Input: dimensioned drawing with shaded views. Units: mm. Origin: part minimum x, y, z. A direction names the side the tool comes from. Coordinates: 2 decimals unless noted, no trailing zeros. Order: outer loops, then holes, each group sorted by start corner. A loop starts at its lowest first (then second) coordinate and runs counter-clockwise, first axis right, second up. Notation, with made-up numbers: (57.5, 5) -> (98.5, 5) arc R20 cw to (98.5, 22) -> close; hole circle Ø1 at (-27.5, 2). An arc over 180 degrees is marked (long way). Answer as CSV lines item,"result".
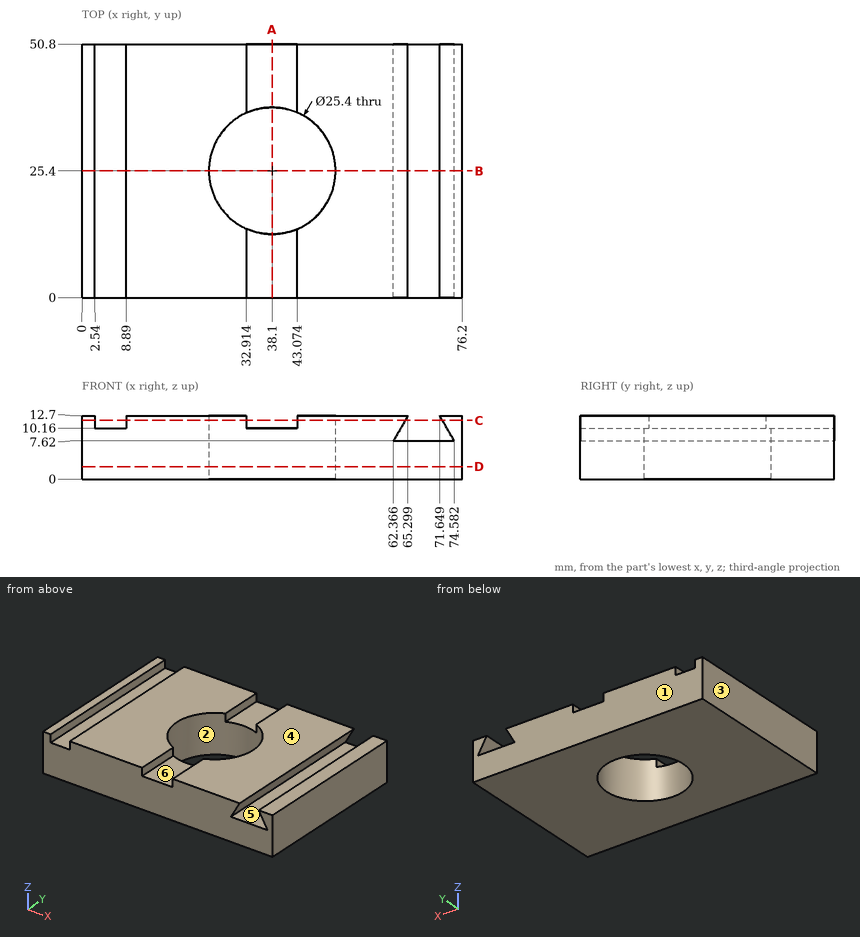
1. Reachability of the marked faces 4, 5 and 6 from +Z, -Z, +X, -X, +Y, -Y: full face, straight path, thin tool, end or side. Return the list, or none.
Findings:
face 4,"+Z, +X, -X, +Y, -Y"
face 5,"+Y, -Y"
face 6,"+Z, +Y, -Y"
2. Cut plane B-B (y = 25.4). Return the cut outline in (x, z).
Findings:
outline,"(0, 0) -> (25.4, 0) -> (25.4, 12.7) -> (8.89, 12.7) -> (8.89, 10.16) -> (2.54, 10.16) -> (2.54, 12.7) -> (0, 12.7) -> close; (50.8, 0) -> (76.2, 0) -> (76.2, 12.7) -> (71.65, 12.7) -> (74.58, 7.62) -> (62.37, 7.62) -> (65.3, 12.7) -> (50.8, 12.7) -> close"
3. Cut plane C-C (z = 11.75). Return the cut outline in (x, y) (1 decimal).
Findings:
outline,"(0, 0) -> (2.5, 0) -> (2.5, 50.8) -> (0, 50.8) -> close; (8.9, 0) -> (32.9, 0) -> (32.9, 13.8) arc R12.7 cw to (32.9, 37) -> (32.9, 50.8) -> (8.9, 50.8) -> close; (43.1, 0) -> (64.8, 0) -> (64.8, 50.8) -> (43.1, 50.8) -> (43.1, 37.1) arc R12.7 cw to (43.1, 13.7) -> close; (72.2, 0) -> (76.2, 0) -> (76.2, 50.8) -> (72.2, 50.8) -> close"
4. Cut plane A-A (x = 38.1). Return the cut outline in (y, z).
Findings:
outline,"(0, 0) -> (12.7, 0) -> (12.7, 10.16) -> (0, 10.16) -> close; (38.1, 0) -> (50.8, 0) -> (50.8, 10.16) -> (38.1, 10.16) -> close"
5. Contact query for flat-ended pins moving along their axis: pin 1 (3 mm diameter, centred on x = 39, y = 41.5, fed in from +Z); pin 2 (10 mm diameter, centred on x = 32.5, y = 27, fed in from -Z). Output: stop coordinate, or through.
Findings:
pin 1,"stops at z = 10.16"
pin 2,"passes through"
6. Mould query, pull axis Y, two halves, no side actions, for the marked faces 1, 2 and 3. Classes: released by +Y, released by -Y, zero draft, split by the parting line, or undercut.
Findings:
face 1,"released by +Y"
face 2,"undercut"
face 3,"zero draft"
7. Ray query, line 1 along Y through (x, z) = (38.1, 5); line 2 along X through (y, z) = (25.4, 4); line 3 along X through (y, z) = (20, 10.5) (1 decimal). Return the intervals inside material, ascending.
Findings:
line 1,"y = 0 to 12.7, 38.1 to 50.8"
line 2,"x = 0 to 25.4, 50.8 to 76.2"
line 3,"x = 0 to 2.5, 8.9 to 26.6, 49.6 to 64, 72.9 to 76.2"
8. Cut plane D-D (z = 2.5). Return the cut outline in (x, y), plus the area to 3 significant figures.
Findings:
outline,"(0, 0) -> (76.2, 0) -> (76.2, 50.8) -> (0, 50.8) -> close; hole circle Ø25.4 at (38.1, 25.4)"
area,"3,360 mm2"
